Work out the finished part from the listing and answer in its coordinate system (mm). A direction names the side the tool comes from. Coordinates: 2 decimals unless noted, no trailing zeros. Write each loop counter-clockwise with the first axis right and the second up, starting at its lowest first coordinate (ties: lowest second). Pieces come first, ordered by that corner, then holes. Notation, with made-up numbers: (-17, 26.5) - (24, 26.5) arc R16 cw to (24, 47.5) - close; hole circle Ø7 at (-1, 20). An arc over 180 degrees is marked (long way). One line per item, written item: value.
```python
from build123d import *

# Parameters (mm, degrees)
F1_R           = 22
F2_DEPTH       = 5
F3_R           = 14
F4_DEPTH       = 355
F4_DEPTH_BACK  = 175
F6_DEPTH       = 40
F7_R           = 10
F9_W           = 4
F9_H           = 175
F10_DEPTH      = 43.001
F10_DEPTH_BACK = 25


with BuildPart() as f2:
    # F1 (on offset) → F2 (new body)
    with BuildSketch(Plane.XY.offset(275)):
        with Locations((154, 0)):
            Circle(F1_R)
    extrude(amount=F2_DEPTH)

    # F3 (on face) → F4 (join, two sides)
    with BuildSketch(Plane.XY.offset(280)) as f4_sk:
        with Locations((154, 0)):
            Circle(F3_R)
    extrude(amount=F4_DEPTH)
    extrude(f4_sk.sketch, amount=-F4_DEPTH_BACK)

    # F5 (on face) → F6 (join)
    with BuildSketch(Plane.XY.offset(635)):
        Polygon((164, 9.7979589711), (163.7979589711, 10), (144.2020410289, 10), (144, 9.8020410289), (144, 9.7979589711), (144.2020410289, -10), (163.8020410289, -10), (164, -9.7979589711), align=None)
    extrude(amount=F6_DEPTH)

    # F7
    f7_edges = [f2.edges().sort_by_distance(p)[0] for p in [
        (140, 0, 105),
    ]]
    fillet(f7_edges, radius=F7_R)

    # F9 (on offset) → F10 (cut, two sides)
    with BuildSketch(Plane.YZ.offset(175)) as f10_sk:
        with Locations((0, 187.5)):
            Rectangle(F9_W, F9_H)
    extrude(amount=-F10_DEPTH, mode=Mode.SUBTRACT)
    extrude(f10_sk.sketch, amount=F10_DEPTH_BACK, mode=Mode.SUBTRACT)


solid = f2.part
```
Item 1: Section B-B, the plane z = 354 is taken. Determine the outline of the cut face in (x, y).
Evaluation:
outline: circle Ø28 at (154, 0)
Item 2: Section A-A, the plane z = 215 is taken. Determine the outline of the cut face in (x, y).
Evaluation:
outline: (140.14, -2) arc R14 ccw to (167.86, -2) - close; (140.14, 2) - (167.86, 2) arc R14 ccw to start
Item 3: Determine the mould class of faces 1 (the face through (164, 0, 655)), 2 (the face through (154, -2, 189)), 3 (the face through (154, 10, 655)) for opening direction Y: +Y half, -Y half, draft (parallel to the pull), parting line (faces both ways), or undercut.
Evaluation:
face 1: draft
face 2: undercut
face 3: +Y half
Item 4: Given pin 1 (2 mm diameter, centred on x = 166.5, y = 0.5, fed in from +Z); pin 2 (2 mm diameter, centred on x = 157.5, y = 7, fed in from -Z); pin 3 (8.5 mm diameter, centred on x = 155.5, z = 219, fed in from +Y), each flat-ended and moving along its own axis, determine where each tip first touches the part or whether it passes through.
Evaluation:
pin 1: stops at z = 635
pin 2: stops at z = 105.41
pin 3: stops at y = 14
Item 5: Consider probe 1 along X at (y, z) = (-9.5, 639); probe 2 along X at (y, z) = (-2, 342.5); probe 3 along Y at (x, z) = (163.5, 155). Determine where each line is inside the solid, lowest interval first.
Evaluation:
probe 1: x = 144.2 to 164
probe 2: x = 140.14 to 167.86
probe 3: y = -10.28 to -2, 2 to 10.28
Item 6: Which of the six approach directions +Z, -Z, +X, -X, +Y, -Y give full straight-line access (tool end or side, diameter ignored) to faces 4 (the face through (154, -14, 196)), 5 (the face through (154, 14, 196)), 6 (the face through (154, -10, 655)), 7 (the face through (154, 2, 189)), 8 (the face through (168.4, 0.3, 280))?
Evaluation:
face 4: -Z, -Y
face 5: -Z, +Y
face 6: +Z, +X, -X, -Y
face 7: -Z, +X, -X
face 8: +Z
